Geometry: final body of the model. Coordinates: model frame, mm. Round coordinates to 2 decimals unless told otherwise and drop trailing zeros. Loops run counter-clockwise (first coordinate to the right, second up) from the corner with the lowest first, then second, coordinate; pieces in that order, holes last. Notation, with made-up numbers: (-20, 54) -> (-1, 54) arc R22 cw to (-1, 84) -> close; hole circle Ø6 at (42.25, -34). An arc over 180 degrees is marked (long way). Answer in a Markdown table with one row per item.
```python
from build123d import *

# Parameters (mm, degrees)
BOSS_EXTRUDE1_DEPTH = 787.4
CAVITY1_START       = 209.393974514
CAVITY1_DEPTH       = 6.25
CUT_EXTRUDE1_DEPTH  = 897.209643935


# Read off the part's stored shape, not the designer's step: Cavity1
with BuildPart() as part:
    # Sketch1 → Boss-Extrude1 (new body)
    with BuildSketch(Plane.XY):
        Polygon((50, 38.1), (46.495004217, 43.274698499), (346.495004217, 246.474698499), (350, 241.3), align=None)
    extrude(amount=BOSS_EXTRUDE1_DEPTH)

    # Cavity1 outline → Cavity1 (cut)
    with BuildSketch(Plane(origin=(0, 0, 0), x_dir=(0.9998289109489032, -0.015681339287170415, -0.009810424501047896), z_dir=(0.018497265493313195, 0.8476202272914186, 0.5302808703467569)).offset(CAVITY1_START)):
        Polygon((42.517859439, -261.403351104), (42.802335744, -261.406643092), (342.564789453, 130.215073828), (188.320866524, 132), (41, 132), (41, -261.385786284), align=None)
    extrude(amount=CAVITY1_DEPTH, mode=Mode.SUBTRACT)

    # Sketch2 → Cut-Extrude1 (cut, through all)
    with BuildSketch(Plane(origin=(-5.470595054, 8.076665927, 0), x_dir=(0.8279517598753687, 0.5607993253555854, 0), z_dir=(-0.5607993253555854, 0.8279517598753687, 0))):
        Polygon((63.112893973, -335.543438937), (425.103993165, -0.59935118), (425.103993165, 0), (62.76404229, 0), (62.76404229, -335.417163823), align=None)
        with BuildLine():
            Line((425.103993165, -787.4), (425.103993165, -786.80064882))
            Line((425.103993165, -786.80064882), (63.112893973, -451.856561063))
            ThreePointArc((63.112893973, -451.856561063), (62.938468131, -451.856470391), (62.76404229, -451.856561063))
            Line((62.76404229, -451.856561063), (62.76404229, -787.4))
            Line((62.76404229, -787.4), (425.103993165, -787.4))
        make_face()
    extrude(amount=-CUT_EXTRUDE1_DEPTH, mode=Mode.SUBTRACT)


solid = part.part
```
Item 1: Pin query (flat end, axial travel): pin 1 Ø12 at (x, z) = (263, 608) entering from -Y; pin 2 Ø5 at (y, z) = (207, 640.5) entering from -X; pin 3 Ø3 at (x, z) = (171.5, 425) entering from -Y. Return the tip coordinate at first contact, or that it passes through.
Answer:
| item | result |
|---|---|
| pin 1 | stops at y = 178.31 |
| pin 2 | stops at x = 284.52 |
| pin 3 | stops at y = 119.38 |
Item 2: Line query: probe 1 along Z at (x, y) = (297, 206); probe 2 along X at (y, z) = (224, 35); probe 3 along Y at (x, z) = (229, 394.5). Output: solid intervals per line, ascending. Write a range as [from, to].
Answer:
| item | result |
|---|---|
| probe 1 | z = [59.52, 727.88] |
| probe 2 | x = [316.81, 324.46] |
| probe 3 | y = [159.34, 166.89] |
Item 3: Cut plane B-B (z = 174). Output: boundary loops of the cut face in (x, y) (3 decimals), then the cut area to 3 significant figures.
Answer:
| item | result |
|---|---|
| outline | (191.334, 141.379) -> (194.839, 136.205) -> (350, 241.3) -> (346.495, 246.475) -> close |
| area | 1,170 mm² |
Item 4: Cut plane A-A (x = 170.5). Output: boundary loops of the cut face in (y, z).
Answer:
| item | result |
|---|---|
| outline | (119.72, 201.2) -> (127.27, 197.28) -> (127.27, 590.12) -> (119.72, 586.2) -> close |
